from build123d import *

# Parameters (mm, degrees)
SKETCH_R     = 29
PAD_DEPTH    = 85
SKETCH001_R  = 17.5
PAD001_DEPTH = 10
FILLET_R     = 4
FILLET001_R  = 4


with BuildPart() as part:
    # Sketch (on XZ_Plane of Origin) → Pad (new body)
    with BuildSketch(Plane.XZ):
        Circle(SKETCH_R)
    extrude(amount=PAD_DEPTH)

    # Sketch001 (on Face3 of Pad) → Pad001 (join)
    with BuildSketch(Plane.XZ.offset(85)):
        Circle(SKETCH001_R)
    extrude(amount=PAD001_DEPTH)

    # Fillet
    fillet_edges = [part.edges().sort_by_distance(p)[0] for p in [
        (-17.5, -85, 0),
    ]]
    fillet(fillet_edges, radius=FILLET_R)

    # Fillet001
    fillet001_edges = [part.edges().sort_by_distance(p)[0] for p in [
        (-17.5, -95, 0),
    ]]
    fillet(fillet001_edges, radius=FILLET001_R)


solid = part.part
Input: part model. Units: mm. Frame: model coordinates. A direction names the side the tool comes from. Coordinates: 2 decimals unless noted, no trailing zeros. Write each loop counter-clockwise with the first axis right and the second up, starting at its lowest first coordinate (ties: lowest second). Pieces come first, ordered by that corner, then holes. Notation, with made-up numbers: M 36.25,-35 L 90.25,-35 A28 cw 90.25,-5 Z; hole C -13.5,62.25 d7. An arc over 180 degrees is marked long. Answer as a JSON object with one key per item and string values. Group by question number.
(1) Section C-C on y = -47. Output: boundary loops of the cut face in (x, z).
(2) Set-up query: faces 1 (the face through (-13.887, -89.986, -10.648)), 2 (the face through (0, 0, 0)). Return all of +Z, -Z, +X, -X, +Y, -Y with unobstructed straight access to the full face (end or side cutting, diameter ignored); none if empty.
(3) Contact query for flat-ended pins moving along their axis: P1, Ø12, axis at x = 0, y = -55, coming from the -Z side; P2, Ø4, axis at y = -21.5, z = 3, coming from the +X side; P3, Ø6, axis at y = -55, z = -3.5, coming from the -X side. Output: stop coordinate, or through.
(4) Section A-A on z = 0. Output: boundary loops of the cut face in (x, y), plus the area to 3 significant figures.
(5) Ray query, line 1 along Z through (x, y) = (1, -37); line 2 along Y through (x, z) = (20, 12). Return the intervals inside material, ascending. Write a range as [from, to].
(6) Section B-B on x = 0. Output: boundary loops of the cut face in (y, z).
Result set:
{
 "1": {"outline": "C 0,0 d58"},
 "2": {"face 1": "-Y", "face 2": "+Z, -Z, +X, -X, +Y"},
 "3": {"P1": "stops at z = -29", "P2": "stops at x = 28.98", "P3": "stops at x = -29"},
 "4": {"outline": "M -29,-85 L -21.5,-85 A4 cw -17.5,-89 L -17.5,-91 A4 ccw -13.5,-95 L 13.5,-95 A4 ccw 17.5,-91 L 17.5,-89 A4 cw 21.5,-85 L 29,-85 L 29,0 L -29,0 Z", "area": "5,280 mm2"},
 "5": {"line 1": "z = [-28.98, 28.98]", "line 2": "y = [-85, 0]"},
 "6": {"outline": "M -95,-13.5 A4 ccw -91,-17.5 L -89,-17.5 A4 cw -85,-21.5 L -85,-29 L 0,-29 L 0,29 L -85,29 L -85,21.5 A4 cw -89,17.5 L -91,17.5 A4 ccw -95,13.5 Z"}
}
